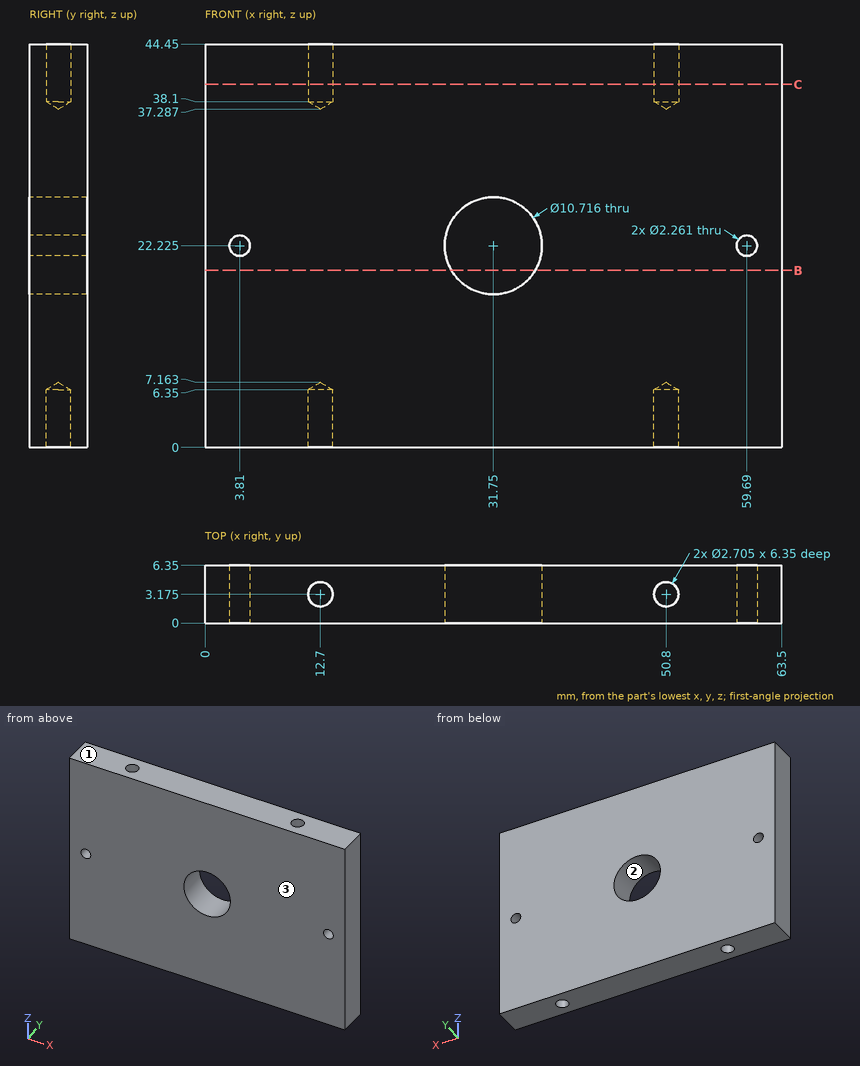
Verification items for this drawing (mm, ordinates from the low corner). Round coordinates to 2 decimals unless told otherwise and drop trailing zeros. Order: outer loops, then holes, each group sorted by start corner. A loop starts at its lowest first (then second) coordinate and runs counter-clockwise, first axis right, second up. Notation, with made-up numbers: (-27.75, 20) - (-22.75, 20) arc R30 ccw to (-22.75, 45) - close; hole circle Ø9 at (-30, 32.5). An arc over 180 degrees is marked (long way). Use CSV: the item, a comma, the result in double quotes. Start each with the question number.
1) Go/stop test with a flat-tipped pin: P1, Ø2, axis at x = 50.8, y = 3.175, coming from the -Z side. Record where the tip stops, or that it passes through.
2) Section check C-C, the plane z = 40. State how many separate pieces and enclosed holes the cut face has, plus the area to 3 significant figures.
3) Mould release check, pull along Z, two halves, no side actions. Record for the marked faces 1, 2 and 3: +Z half, -Z half, draft (parallel to the pull), parting line (faces both ways), or undercut.
4) Section check B-B, the plane z = 19.5. Record the cut outline in (x, y), plus the area to 3 significant figures.
5) Thickness scan on L1, parallel to Y at x = 50.8, z = 3.75; L2, parallel to X at y = 3.5, z = 38.5; L3, parallel to Z at x = 35.5, y = 1.25. Record the ranges inside material, lowest first.
Answers:
1,P1,"stops at z = 6.56"
2,separate pieces,"1"
2,enclosed holes,"2"
2,area,"392 mm²"
3,face 1,"+Z half"
3,face 2,"undercut"
3,face 3,"draft"
4,outline,"(0, 0) - (27.14, 0) - (27.14, 6.35) - (0, 6.35) - close; (36.36, 0) - (63.5, 0) - (63.5, 6.35) - (36.36, 6.35) - close"
4,area,"345 mm²"
5,L1,"y = 0 to 1.82, 4.53 to 6.35"
5,L2,"x = 0 to 11.39, 14.01 to 49.49, 52.11 to 63.5"
5,L3,"z = 0 to 18.4, 26.05 to 44.45"
